Autodesk Inventor part; units mm, degrees
ref_plane "YZ Plane" through (0, 0, 0) normal (1, 0, 0) x (0, 1, 0)
ref_plane "XZ Plane" through (0, 0, 0) normal (0, 1, 0) x (-1, 0, 0)
ref_plane "XY Plane" through (0, 0, 0) normal (0, 0, 1) x (1, 0, 0)
sketch "Sketch1" plane through (0, 0, 0) normal (0, 0, 1) x (1, 0, 0)
  line L0 (18.6455, 5.0782) -> (18.6456, 5.0782)
  circle A0 centre (26.2482, -10.4107) radius 8.7948
  line L1 (39.4932, 48.3268) -> (39.4932, -31.0482)
  line L2 (13.0032, -31.0482) -> (13.0032, 48.3268)
  line L3 (13.0032, 48.3268) -> (39.4932, 48.3268)
  line L4 (39.4932, -31.0482) -> (13.0032, -31.0482)
  circle A1 centre (26.2471, -24.96) radius 1.5875
  point P0 (0, 0)
  dimension "d0" = 17.5895
  dimension "d3" = 26.49
  dimension "d4" = 13.245
  dimension "d5" = 58.7375
  dimension "d6" = 79.375
  dimension "d15" = 3.175
  dimension "d25" = 26.49
  dimension "d26" = 13.2461
extrude "Extrusion1" add sketch "Sketch1" against normal blind 5.6134 contours L1 L4 L2 L3 | A1
sketch "Sketch2" plane through (0, 0, 0) normal (0, 0, 1) x (1, 0, 0)
  line L0 (13.0032, 48.3268) -> (39.4932, 48.3268)
  circle A0 centre (26.2482, 41.9768) radius 1.6002
  point P0 (0, 0)
  point P1 (0, 0)
  dimension "d10" = 3.2004
  dimension "d12" = 6.35
extrude "Extrusion2" cut sketch "Sketch2" against normal blind 5.6134
sketch "Sketch3" plane through (0, 0, 0) normal (0, 0, 1) x (1, 0, 0)
  circle A0 centre (26.2482, -10.4107) radius 8.7947
  circle A1 centre (26.2471, -26.3619) radius 1.7272
  line L0 (39.4932, 48.3268) -> (39.4932, -31.0482)
  point P0 (0, 0)
  dimension "d17" = 3.4544
  dimension "d18" = 15.9512
  dimension "d27" = 13.2461
extrude "Extrusion3" cut sketch "Sketch3" against normal blind 5.6134 contours A1
fillet "Fillet1" radius 6.35 2 edges at (13.0032, 48.3268, -2.8067) (39.4932, 48.3268, -2.8067)
sketch "Sketch5" plane through (0, 0, -5.6134) normal (0, 0, -1) x (-1, 0, 0)
  circle A0 centre (-26.2482, -10.4107) radius 8.7947
  circle A1 centre (-26.2482, -10.4107) radius 6.9215
  point P0 (0, 0)
  dimension "d28" = 13.843
extrude "Extrusion5" add sketch "Sketch5" against normal blind 1.5875
properties part number "Lidar Sensor Case v4 Piece 1"
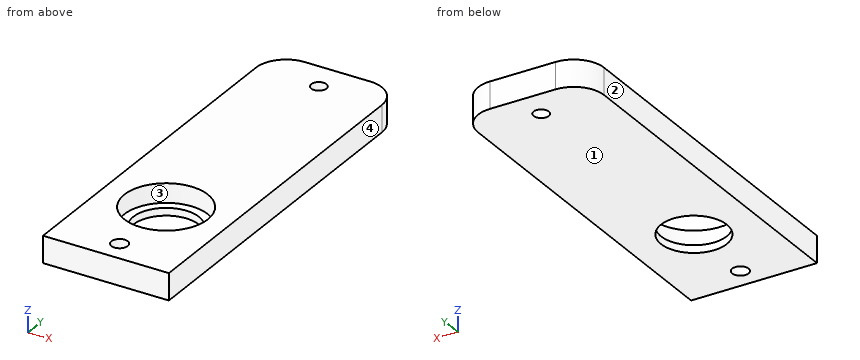
Input: part model. Units: mm. Frame: model coordinates. Face numbers are marked on the shaded views. Give positions to 0.01 mm unless a question says otherwise; leave off trailing zeros. Order: outer loops, then holes, each group sorted by start corner. A loop starts at its lowest first (then second) coordinate and runs counter-clockwise, first axis right, second up. Notation, with made-up numbers: M 1.5,-2.5 L 52.5,-2.5 A21 ccw 52.5,28.5 Z; hole C 48.25,-1 d3. An arc over 180 degrees is marked long. One line per question, with ' | ' between items. Start each with the question number.
1. Section query B-B (z = -2.15). Return the cut outline in (x, y), and give its area (3 significant figures).
2. Material intervals for probe 1 along Y at (x, z) = (25.5, -2.45); probe 2 along Y at (x, z) = (26.75, -4.95); probe 3 along Y at (x, z) = (30.75, -2.9), sorted ascending. Write a range as [from, to].
3. Section query C-C (x = 23.75). Return the cut outline in (y, z).
4. Section query D-D (x = 37.25). Return the cut outline in (y, z).
5. Pull-direction query (X, two-part tool) for the marked faces 1, 2, 3 and 4; classes: released by +X, released by -X, zero draft, split by the parting line, or undercut.
6. First-contact query: pin 1 Ø2.5 at (x, y) = (26.25, 41.98) entering from -Z; pin 2 Ø4 at (x, y) = (29.5, -6) entering from +Z. Flat tips, straight axial feed; report the tip coordinate or a pass-through.
7. Section query A-A (x = 20.5). Return the cut outline in (y, z), and give its area (3 significant figures).
Here are the results:
1) outline: M 13,-31.05 L 39.49,-31.05 L 39.49,41.98 A6.35 ccw 33.14,48.33 L 19.35,48.33 A6.35 ccw 13,41.98 Z; hole C 26.25,-10.41 d17.59; hole C 26.25,-26.36 d3.45; hole C 26.25,41.98 d3.2 | area: 1,820 mm²
2) probe 1: [-31.05, -27.92], [-24.8, -19.17], [-1.65, 40.56], [43.39, 48.33] | probe 2: [-31.05, -28.01], [-24.71, -17.31], [-3.51, 40.46], [43.5, 48.33] | probe 3: [-31.05, -17.97], [-2.86, 48.33]
3) outline: M -31.05,-5.61 L -16.87,-5.61 L -16.87,-4.03 L -18.84,-4.03 L -18.84,0 L -31.05,0 Z; M -3.96,-5.61 L 48.33,-5.61 L 48.33,0 L -1.98,0 L -1.98,-4.03 L -3.96,-4.03 Z
4) outline: M -31.05,-5.61 L 46.82,-5.61 L 46.82,0 L -31.05,0 Z
5) face 1: zero draft | face 2: released by -X | face 3: undercut | face 4: released by +X
6) pin 1: through | pin 2: z = -4.03
7) outline: M -31.05,-5.61 L -14.27,-5.61 L -14.27,-4.03 L -17.07,-4.03 L -17.07,0 L -31.05,0 Z; M -6.56,-5.61 L 48.33,-5.61 L 48.33,0 L -3.75,0 L -3.75,-4.03 L -6.56,-4.03 Z | area: 380 mm²
